Autodesk Inventor part; units mm, degrees
ref_plane "YZ Plane" through (0, 0, 0) normal (1, 0, 0) x (0, 1, 0)
ref_plane "XZ Plane" through (0, 0, 0) normal (0, 1, 0) x (-1, 0, 0)
ref_plane "XY Plane" through (0, 0, 0) normal (0, 0, 1) x (1, 0, 0)
sketch "Sketch1" plane through (0, 0, 0) normal (0, 1, 0) x (-1, 0, 0)
  line L0 (-3.5, -3.5) -> (0.1946, -3.5) construction
  arc A0 (-5.4544, -2.5) -> (3.5, 4.8734) centre (0, 0) ccw
  line L1 (0, -6) -> (0, -7)
  line L2 (0, -7) -> (1.3359, -5.4079)
  line L3 (0, -7) -> (2.0783, -7) construction
  line L4 (0, -7) -> (-1.4433, -5.2799)
  line L5 (0, -7) -> (2.2454, -7) construction
  circle A1 centre (0, 0) radius 6
  arc A2 (-0.4195, -6.5) -> (0.4195, -6.5) centre (0, -6.228) ccw
  line L6 (2.5, 3.5) -> (-2.5, 3.5)
  line L7 (-2.5, 3.5) -> (-2.5, -3.5)
  line L8 (-2.5, -3.5) -> (2.5, -3.5)
  line L9 (2.5, -3.5) -> (2.5, 3.5)
  point P0 (-204.25, 70)
  point P1 (-7, 0)
  point P2 (-200.75, 67.5)
  point P3 (-0.8955, -5.9328)
  point P4 (0.8955, -5.9328)
  point P5 (-0.3407, -6.594)
  point P6 (0.3407, -6.594)
  point P7 (3.5, 4.8734)
  point P8 (-5.4544, -2.5)
  dimension "d0" = 1
  dimension "d1" = 50
  dimension "d2" = 130
  dimension "d3" = 0.5
  dimension "d6" = 7
  dimension "d7" = 5
  dimension "d8" = 3.5
  dimension "d9" = 2.5
extrude "Extrusion1" add sketch "Sketch1" along normal blind 6 contours A0 A1
sketch "Sketch2" plane through (0, 6, 0) normal (0, 1, 0) x (1, 0, 0)
  arc A0 (-5.4544, -2.5) -> (3.5, 4.8734) centre (0, 0) ccw
  line L0 (0, -6) -> (0, -7)
  line L1 (0, -7) -> (1.3359, -5.4079)
  line L2 (0, -7) -> (2.0783, -7) construction
  line L3 (0, -7) -> (-1.4433, -5.2799)
  line L4 (0, -7) -> (2.2454, -7) construction
  circle A1 centre (0, 0) radius 6
  arc A2 (-0.4195, -6.5) -> (0.4195, -6.5) centre (0, -6.228) ccw
  point P0 (-200.75, 67.5)
  point P1 (-0.8955, -5.9328)
  point P2 (0.8955, -5.9328)
  point P3 (-0.3407, -6.594)
  point P4 (0.3407, -6.594)
  point P5 (-0.3407, -6.594)
  point P6 (0.3407, -6.594)
  point P7 (0.8955, -5.9328)
  point P8 (-0.8955, -5.9328)
  dimension "d12" = 1
  dimension "d13" = 50
  dimension "d14" = 130
  dimension "d15" = 0.5
extrude "Extrusion2" add sketch "Sketch2" against normal blind 2 contours L3 A0 L0 A2 | L1 A2 L0 A0
pattern_circular "Circular Pattern1" count 21 over 360 about axis through (0, 0, 0) along (0, 1, 0) of "Extrusion2"
sketch "Sketch3" plane through (0, 6, 0) normal (0, 1, 0) x (1, 0, 0)
  circle A0 centre (0, 0) radius 7.9508
  circle A1 centre (0, 0) radius 4.6059
extrude "Extrusion3" add sketch "Sketch3" against normal blind 6
sketch "Sketch4" plane through (0, 6, 0) normal (0, 1, 0) x (1, 0, 0)
  circle A0 centre (0, 0) radius 7.9508
  line L0 (-7.9508, 0) -> (-7.3848, 2.9463)
  line L1 (-7.9508, 0) -> (-10.7252, 0.533)
  line L2 (-7.3848, 2.9463) -> (-10.1592, 3.4793)
  line L3 (-7.6678, 1.4731) -> (-9.6319, 1.8505)
  line L4 (-7.9508, 0) -> (-9.6319, 1.8505)
  line L5 (-7.3848, 2.9463) -> (-9.6319, 1.8505)
  arc A1 (-8.5083, 2.3984) -> (-8.7914, 0.9252) centre (-8.1829, 1.5721) ccw
  point P0 (-8.6335, 2.3373)
  point P1 (-8.885, 1.0283)
extrude "Extrusion4" add sketch "Sketch4" against normal blind 6 contours L4 L3 A1 | L5 A0 L3 A1 | L4 A1 L3 A0 | A1 L3 L5
pattern_circular "Circular Pattern2" count 16 over 360 about axis through (0, 6, 0) along (0, -1, 0) of "Extrusion4"
sketch "Sketch5" plane through (0, 6, 0) normal (0, 1, 0) x (1, 0, 0)
  point P0 (0, 0)
equation "\"BendRadius\" = Thickness"
equation "\"BendReliefWidth\" = Thickness"
equation "\"BendReliefDepth\" = 0.5 * Thickness"
equation "\"CornerReliefSize\" = 4 * Thickness"
equation "\"MinimumRemnant\" = 2 * Thickness"
equation "\"TransitionRadius\" = BendRadius"
equation "\"JacobiRadiusSize\" = BendRadius"
equation "\"GapSize\" = Thickness"
properties part number "modelGateGear"
Design review of the part built by this model. Coordinates are the model's own, in mm. A direction names the side the tool comes from. Round coordinates to 2 decimals unless told otherwise and drop trailing zeros. Loops run counter-clockwise (first coordinate to the right, second up) from the corner with the lowest first, then second, coordinate; pieces in that order, holes last. Notation, with made-up numbers: M 51.5,33.25 L 88.5,33.25 A5 cw 88.5,40.25 Z; hole C -2,-23.5 d11. An arc over 180 degrees is marked long. Answer as a JSON object with one key per item and string values.
Item 1: The part is to be moulded in two halves that separate along Z. For faces 1 (the flat face through (4.2, 3.04, -7.76)), 2 (the flat face through (-2.5, 3, 0)), 3 (the flat face through (2.5, 3, 0)), 4 (the flat face through (4, 6, 0)), say which applies: pulls with the +Z half, pulls with the -Z half, needs draft (parallel to the pull), parting line crosses it, or undercut.
Answer sheet:
{"face 1": "pulls with the -Z half", "face 2": "undercut", "face 3": "undercut", "face 4": "needs draft"}
Item 2: We need section A-A on x = 8.5. Give the boundary of the cut face in (y, z).
Answer sheet:
{"outline": "M 0,-2.5 L 6,-2.5 L 6,-0.73 L 0,-0.73 Z; M 0,0.6 L 6,0.6 L 6,2.4 L 0,2.4 Z"}
Item 3: Clearance check with flat-ended pins moving along their axes: P1, Ø2.5, axis at x = 0, y = 4, coming from the -Z side; P2, Ø1.5, axis at y = 2, z = -0.5, coming from the -X side. State where each tip first meets the part, or that it passes through.
Answer sheet:
{"P1": "stops at z = -9.09", "P2": "stops at x = -9.09"}
Item 4: We need section D-D on x = 6. Give the boundary of the cut face in (y, z), and give its area (3 significant figures).
Answer sheet:
{"outline": "M 0,-5.6 L 6,-5.6 L 6,5.53 L 0,5.53 Z", "area": "66.8 mm^2"}
Item 5: Machinability: for faces 5 (the flat face through (4.304, 3.042, 7.707)), 6 (the flat face through (0.91, 3.04, -8.78)), 7 (the flat face through (-7.707, 3.042, 4.304)), which of the approach directions +Z, -Z, +X, -X, +Y, -Y give a long, thin tool a straight path to every point of the face, cutting with its end or side? Answer none if there is none.
Answer sheet:
{"face 5": "+Z, +Y, -Y", "face 6": "-Z, +Y, -Y", "face 7": "-X, +Y, -Y"}
Item 6: We need section C-C on z = -6. Give the boundary of the cut face in (x, y).
Answer sheet:
{"outline": "M -5.6,0 L 5.53,0 L 5.53,6 L -5.6,6 Z"}
Item 7: Wall thickness on L1, parallel to X at y = 0.75, z = -8.75; L2, parallel to Z at x = -2, y = 0.8; L3, parallel to X at y = 3.05, z = -0.5: over which ranges is each line inside the solid? List them lowest first. Write a range as from..to.
Answer sheet:
{"L1": "x = -2.38..-1.01, 0.88..2.28", "L2": "z = -9.56..-3.5, 3.5..9.33", "L3": "x = -8.41..-2.5, 2.5..8.3"}
Item 8: We need section B-B on z = -1.5. Give the boundary of the cut face in (x, y), and give its area (3 significant figures).
Answer sheet:
{"outline": "M -9.31,0 L -2.5,0 L -2.5,6 L -9.31,6 Z; M 2.5,0 L 9.19,0 L 9.19,6 L 2.5,6 Z", "area": "81.0 mm^2"}
